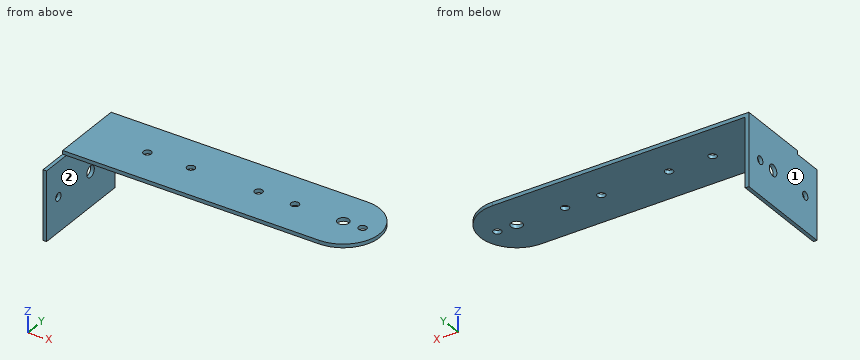
from build123d import *

# Parameters (mm, degrees)
BOSS_EXTRUDE1_DEPTH = 1.59
SKETCH2_W           = 1.59
SKETCH2_H           = 45
BOSS_EXTRUDE2_DEPTH = 30.41
SKETCH3_R           = 1.75
SKETCH3_R_2         = 2.5
CUT_EXTRUDE1_DEPTH  = 121.32593486
SKETCH4_R           = 2.5
SKETCH4_R_2         = 1.75
CUT_EXTRUDE2_DEPTH  = 30.41


with BuildPart() as part:
    # Sketch1 → Boss-Extrude1 (new body)
    with BuildSketch(Plane.XY):
        with BuildLine():
            Line((0, 16), (-112.75, 16))
            Line((-112.75, 16), (-112.75, -16))
            Line((-112.75, -16), (0, -16))
            ThreePointArc((0, -16), (16, 0), (0, 16))
        make_face()
    extrude(amount=BOSS_EXTRUDE1_DEPTH)

    # Sketch2 → Boss-Extrude2 (add)
    with BuildSketch(Plane(origin=(0, 0, 0), x_dir=(-1, 0, 0), z_dir=(0, 0, -1))):
        with Locations((111.955, -6.5)):
            Rectangle(SKETCH2_W, SKETCH2_H)
    extrude(amount=BOSS_EXTRUDE2_DEPTH)

    # Sketch3 → Cut-Extrude1 (cut, through all)
    with BuildSketch(Plane(origin=(0, 0, 0), x_dir=(-1, 0, 0), z_dir=(0, 0, -1))):
        with Locations((86.16, 0)):
            Circle(SKETCH3_R)
        with Locations((37.25, 0)):
            Circle(SKETCH3_R)
        with Locations((67, 0)):
            Circle(SKETCH3_R)
        with Locations((-8.5, 0)):
            Circle(SKETCH3_R)
        Circle(SKETCH3_R_2)
        with Locations((21.25, 0)):
            Circle(SKETCH3_R)
    extrude(amount=-CUT_EXTRUDE1_DEPTH, mode=Mode.SUBTRACT)

    # Sketch4 → Cut-Extrude2 (cut)
    with BuildSketch(Plane.ZY.offset(112.75)):
        with Locations((-15.205, 0)):
            Circle(SKETCH4_R)
        with Locations((-15.205, 8.5)):
            Circle(SKETCH4_R_2)
        with Locations((-15.205, -21.25)):
            Circle(SKETCH4_R_2)
    extrude(amount=-CUT_EXTRUDE2_DEPTH, mode=Mode.SUBTRACT)


solid = part.part
Geometry: final body of the model. Coordinates: model frame, mm. Face numbers are marked on the shaded views. A direction names the side the tool comes from. Round coordinates to 2 decimals unless told otherwise and drop trailing zeros. Order: outer loops, then holes, each group sorted by start corner. A loop starts at its lowest first (then second) coordinate and runs counter-clockwise, first axis right, second up. Notation, with made-up numbers: (-18.75, 27.5) -> (11.25, 27.5) arc R12 ccw to (11.25, 46.5) -> close; hole circle Ø9 at (63.25, -8.5). An arc over 180 degrees is marked (long way). Put each result on its own line as item: value. Start each with the question number.
Q1. Section A-A on y = 0. Give the number of separate pieces and of enclosed holes in the cut face, and give its area (3 significant figures).
Q2. Section C-C on y = 8.5. Return the cut outline in (x, z) (3 decimals).
Q3. Section B-B on x = -86.16. Return the cut outline in (y, z), and give its area (3 significant figures).
Q4. Reachability of the marked faces 1 and 2 from +Z, -Z, +X, -X, +Y, -Y: full face, straight path, thin tool, end or side. Return the list, or none.
Q5. First-contact query: pin 1 (4.5 mm diameter, centred on x = -86.16, y = 0, fed in from -Z); pin 2 (3 mm diameter, centred on x = -21.25, y = 0, fed in from -Z); pin 3 (1.7 mm diameter, centred on x = -111.5, y = -22, fed in from +Z); pin 4 (5.5 mm diameter, centred on y = -21.25, z = -15.205, fed in from +X). Flat tips, straight axial feed; report the tip coordinate or a pass-through.
Q6. Line query: probe 1 along Y at (x, z) = (-37.25, 0.7); probe 2 along X at (y, z) = (-12.5, -21.5); probe 3 along Z at (x, y) = (-24.5, 5). Output: solid intervals per line, ascending.
Q7. Section D-D on z = -20. Return the cut outline in (x, y).
Ans:
1. separate pieces: 8
1. enclosed holes: 0
1. area: 209 mm2
2. outline: (-112.75, -30.41) -> (-111.16, -30.41) -> (-111.16, -16.955) -> (-112.75, -16.955) -> close; (-112.75, -13.455) -> (-111.16, -13.455) -> (-111.16, 0) -> (13.555, 0) -> (13.555, 1.59) -> (-112.75, 1.59) -> close
3. outline: (-16, 0) -> (-1.75, 0) -> (-1.75, 1.59) -> (-16, 1.59) -> close; (1.75, 0) -> (16, 0) -> (16, 1.59) -> (1.75, 1.59) -> close
3. area: 45.3 mm2
4. face 1: +Z, -Z, -X, +Y, -Y
4. face 2: -Z, +X, +Y, -Y
5. pin 1: stops at z = 0
5. pin 2: passes through
5. pin 3: stops at z = 0
5. pin 4: stops at x = -111.16
6. probe 1: y = -16 to -1.75, 1.75 to 16
6. probe 2: x = -112.75 to -111.16
6. probe 3: z = 0 to 1.59
7. outline: (-112.75, -29) -> (-111.16, -29) -> (-111.16, 16) -> (-112.75, 16) -> close
